from build123d import *

# Parameters (mm, degrees)
SKETCH_1_W      = 16
SKETCH_1_H      = 16
SKETCH_1_W_2    = 12
SKETCH_1_H_2    = 12
EXTRUDE_1_DEPTH = 2
SKETCH_2_W      = 2
SKETCH_2_H      = 2
EXTRUDE_2_DEPTH = 12
SKETCH_3_W      = 2
SKETCH_3_H      = 2
SKETCH_3_W_2    = 12
SKETCH_3_H_2    = 1.99
EXTRUDE_3_DEPTH = 2
FILLET_1_R      = 1
FILLET_2_R      = 1


with BuildPart() as part:
    # 草图1 → 凸台-拉伸1 (new body)
    with BuildSketch(Plane(origin=(0, 0, 0), x_dir=(0, 0, -1), z_dir=(1, 0, 0))):
        with Locations((8, -8)):
            Rectangle(SKETCH_1_W, SKETCH_1_H)
        with Locations((8, -8)):
            Rectangle(SKETCH_1_W_2, SKETCH_1_H_2, mode=Mode.SUBTRACT)
    extrude(amount=EXTRUDE_1_DEPTH)

    # 草图2 → 凸台-拉伸2 (add)
    with BuildSketch(Plane(origin=(2, 0, 0), x_dir=(0, 0, -1), z_dir=(1, 0, 0))):
        with Locations((5.666666, -1)):
            Rectangle(SKETCH_2_W, SKETCH_2_H)
        with Locations((1, -1)):
            Rectangle(SKETCH_2_W, SKETCH_2_H)
        with Locations((10.333332, -1)):
            Rectangle(SKETCH_2_W, SKETCH_2_H)
        with Locations((15, -1)):
            Rectangle(SKETCH_2_W, SKETCH_2_H)
        with Locations((1, -5.67)):
            Rectangle(SKETCH_2_W, SKETCH_2_H)
        with Locations((1, -10.34)):
            Rectangle(SKETCH_2_W, SKETCH_2_H)
        with Locations((1, -15)):
            Rectangle(SKETCH_2_W, SKETCH_2_H)
        with Locations((10.33, -15)):
            Rectangle(SKETCH_2_W, SKETCH_2_H)
        with Locations((15, -15)):
            Rectangle(SKETCH_2_W, SKETCH_2_H)
        with Locations((5.66, -15)):
            Rectangle(SKETCH_2_W, SKETCH_2_H)
        with Locations((15, -10.33)):
            Rectangle(SKETCH_2_W, SKETCH_2_H)
        with Locations((15, -5.66)):
            Rectangle(SKETCH_2_W, SKETCH_2_H)
    extrude(amount=EXTRUDE_2_DEPTH)

    # 草图3 → 凸台-拉伸3 (add)
    with BuildSketch(Plane(origin=(14, 0, 0), x_dir=(0, 0, -1), z_dir=(1, 0, 0))):
        with Locations((1, -1)):
            Rectangle(SKETCH_3_W, SKETCH_3_H)
        Polygon((2, -2), (0, -2), (0, -16), (2, -16), (2, -14), (2, -11.33), (2, -9.34), (2, -6.66), (2, -4.67), align=None)
        Polygon((2, -14), (2, -16), (16, -16), (16, -14), (14, -14), align=None)
        Polygon((16, 0), (14, 0), (14, -2), (14, -4.67), (14, -6.66), (14, -9.34), (14, -11.33), (14, -14), (16, -14), align=None)
        with Locations((8, -1)):
            Rectangle(SKETCH_3_W_2, SKETCH_3_H)
        with Locations((8, -5.665)):
            Rectangle(SKETCH_3_W_2, SKETCH_3_H_2)
        with Locations((8, -10.335)):
            Rectangle(SKETCH_3_W_2, SKETCH_3_H_2)
    extrude(amount=EXTRUDE_3_DEPTH)

    # 圆角1
    fillet_1_edges = [part.edges().sort_by_distance(p)[0] for p in [
        (16, -16, -8),
        (16, -8, -16),
        (16, 0, -8),
        (16, -8, 0),
        (8, 0, 0),
        (8, 0, -16),
        (8, -16, -16),
        (8, -16, 0),
    ]]
    fillet(fillet_1_edges, radius=FILLET_1_R)

    # 圆角2
    fillet_2_edges = [part.edges().sort_by_distance(p)[0] for p in [
        (8, -16, -2),
        (8, -14, 0),
        (8, -16, -9.33),
        (8, -16, -11.33),
        (8, -16, -4.66),
        (8, -16, -6.66),
        (8, -11.33, -16),
        (8, -9.33, -16),
        (8, -6.66, -16),
        (8, -4.66, -16),
        (8, -2, 0),
        (8, 0, -2),
        (8, -14, -16),
        (8, -16, -14),
        (8, 0, -6.666666),
        (8, 0, -4.666666),
        (8, 0, -11.333332),
        (8, 0, -9.333332),
        (8, 0, -14),
        (8, -2, -16),
        (8, -4.67, 0),
        (8, -6.67, 0),
        (8, -9.34, 0),
        (8, -11.34, 0),
    ]]
    fillet(fillet_2_edges, radius=FILLET_2_R - 0.0001)  # a hair under: the kernel refuses the full size


solid = part.part
Input: part model. Units: mm. Frame: model coordinates. A direction names the side the tool comes from. Give positions to 0.01 mm unless a question says otherwise; leave off trailing zeros. Order: outer loops, then holes, each group sorted by start corner. A loop starts at its lowest first (then second) coordinate and runs counter-clockwise, first axis right, second up. Notation, with made-up numbers: (-36.75, 24) - (15.25, 24) arc R14 cw to (15.25, 38) - close; hole circle Ø10 at (57, 47). An arc over 180 degrees is marked (long way). Answer as a JSON object with one key per item and string values. Group by question number.
Q1. Cut plane A-A, the plane y = -12. Output: boundary loops of the cut face in (x, z), then the cut area to 3 significant figures.
Q2. Line query: probe 1 along Y at (x, z) = (14.25, -10.75); probe 2 along Z at (x, y) = (1.75, -10); probe 3 along Z at (x, y) = (6.25, -1.5). Output: solid intervals per line, ascending.
Q3. Set-up query: faces 1 (the face through (7.9, -1.5, -6.667)), 2 (the face through (7.9, -2, -1.5)), 3 (the face through (6, -11, -2)). Return all of +Z, -Z, +X, -X, +Y, -Y with unobstructed straight access to the full face (end or side cutting, diameter ignored); none if empty.
Q4. Cut plane B-B, the plane z = -8.25. Output: boundary loops of the cut face in (x, y).
Q5. First-contact query: pin 1 Ø6 at (x, z) = (11.5, -5) entering from +Y; pin 2 Ø0.6 at (y, z) = (-10.5, -5.5) entering from -X; pin 3 Ø0.8 at (x, y) = (6.5, -14.5) entering from +Z (3 decimals). Flat tips, straight axial feed; report the tip coordinate or a pass-through.
Q6. Mould query, pull axis Z, two halves, no side actions, for faces 4 (the face through (8.084, -15.715, -14.301)), 5 (the face through (7.395, -0.301, -0.285)), 6 (the face through (14, -8, -15)). Classes: pulls with the +Z half, pulls with the -Z half, needs draft (parallel to the pull), parting line crosses it, or undercut.
Q7. Cut plane D-D, the plane x = 6.5. Count the separate pieces of the cut face and the enclosed holes in it, then the cut area to 3 significant figures.
Q8. Cut plane C-C, the plane z = -6.25. Output: boundary loops of the cut face in (x, y).
Results:
{
 "1": {"outline": "(0, -16) - (2, -16) - (2, -14) - (0, -14) - close; (0, -2) - (2, -2) - (2, 0) - (0, 0) - close; (14, -16) - (15, -16) arc R1 ccw to (16, -15) - (16, -14) - (14, -14) - close; (14, -2) - (16, -2) - (16, -1) arc R1 ccw to (15, 0) - (14, 0) - close", "area": "15.6 mm^2"},
 "2": {"probe 1": "-16 to -14, -11.33 to -9.34, -6.66 to -4.67, -2 to 0", "probe 2": "-16 to -14, -2 to 0", "probe 3": "-15.87 to -14, -11.33 to -9.33, -6.67 to -4.67, -2 to -0.13"},
 "3": {"face 1": "+Y, -Y", "face 2": "+Z, -Z", "face 3": "-X"},
 "4": {"outline": "(0, -16) - (2, -16) - (2, -14) - (0, -14) - close; (0, -2) - (2, -2) - (2, 0) - (0, 0) - close; (14, -16) - (15, -16) arc R1 ccw to (16, -15) - (16, -14) - (14, -14) - close; (14, -11.33) - (16, -11.33) - (16, -9.34) - (14, -9.34) - close; (14, -6.66) - (16, -6.66) - (16, -4.67) - (14, -4.67) - close; (14, -2) - (16, -2) - (16, -1) arc R1 ccw to (15, 0) - (14, 0) - close"},
 "5": {"pin 1": "y = 0", "pin 2": "x = 14", "pin 3": "z = -0.005"},
 "6": {"face 4": "undercut", "face 5": "pulls with the +Z half", "face 6": "needs draft"},
 "7": {"separate pieces": "12", "enclosed holes": "0", "area": "42.0 mm^2"},
 "8": {"outline": "(0, -16) - (2, -16) - (2, -15.81) - (14, -15.81) - (14, -16) - (15, -16) arc R1 ccw to (16, -15) - (16, -14) - (0, -14) - close; (0, -2) - (16, -2) - (16, -1) arc R1 ccw to (15, 0) - (14, 0) - (14, -0.19) - (2, -0.19) - (2, 0) - (0, 0) - close; (14, -11.33) - (16, -11.33) - (16, -9.34) - (14, -9.34) - close; (14, -6.66) - (16, -6.66) - (16, -4.67) - (14, -4.67) - close"}
}
